Autodesk Inventor part; units mm, degrees
ref_plane "YZ Plane" through (0, 0, 0) normal (1, 0, 0) x (0, 1, 0)
ref_plane "XZ Plane" through (0, 0, 0) normal (0, 1, 0) x (-1, 0, 0)
ref_plane "XY Plane" through (0, 0, 0) normal (0, 0, 1) x (1, 0, 0)
sketch "Sketch1" plane through (0, 0, 0) normal (0, 0, 1) x (1, 0, 0)
  line L0 (0, 0) -> (25.4, 0)
  line L1 (25.4, 0) -> (25.4, 50.8)
  line L2 (25.4, 50.8) -> (0, 50.8)
  line L3 (0, 50.8) -> (0, 0)
  line L4 (1.5875, 49.2125) -> (23.8125, 49.2125)
  line L5 (23.8125, 49.2125) -> (23.8125, 1.5875)
  line L6 (23.8125, 1.5875) -> (1.5875, 1.5875)
  line L7 (1.5875, 1.5875) -> (1.5875, 49.2125)
  dimension "d0" = 25.4
  dimension "d1" = 50.8
  dimension "d2" = 1.5875
extrude "Extrusion1" add sketch "Sketch1" along normal blind 76.2
sketch "Sketch2" plane through (25.4, 0, 0) normal (1, 0, 0) x (0, 0, -1)
  circle A0 centre (-38.1, 25.4) radius 7.9375
  point P0 (0, 0)
  dimension "d5" = 15.875
extrude "Extrusion2" cut sketch "Sketch2" against normal blind 4.7625
sketch "Sketch3" plane through (0, 0, 0) normal (-1, 0, 0) x (0, 0, 1)
  circle A0 centre (38.1, 25.4) radius 7.9375
  circle A1 centre (38.1, 25.4) radius 6.35
  point P0 (0, 0)
  dimension "d8" = 12.7
extrude "Extrusion3" cut sketch "Sketch3" against normal blind 4.7625 contours A1
sketch "Sketch4" plane through (0, 0, 0) normal (-1, 0, 0) x (0, 0, 1)
  line L0 (0, 1.5875) -> (0, 49.2125) construction
  line L1 (0, 25.4) -> (12.7, 25.4) construction
  line L2 (12.7, 25.4) -> (63.5, 25.4) construction
  circle A0 centre (12.7, 25.4) radius 2.5797
  circle A1 centre (63.5, 25.4) radius 2.5797
  point P0 (0, 0)
  dimension "d11" = 12.7
  dimension "d12" = 50.8
  dimension "d13" = 5.1594
extrude "Extrusion4" cut sketch "Sketch4" against normal blind 55.5625
sketch "Sketch5" plane through (0, 50.8, 0) normal (0, 1, 0) x (1, 0, 0)
  line L0 (23.8125, 0) -> (1.5875, 0) construction
  line L1 (12.7, 0) -> (12.7, -12.7) construction
  line L2 (12.7, -12.7) -> (12.7, -63.5) construction
  circle A0 centre (12.7, -12.7) radius 2.5797
  circle A1 centre (12.7, -63.5) radius 2.5797
  point P0 (0, 0)
  dimension "d16" = 12.7
  dimension "d17" = 50.8
  dimension "d18" = 5.1594
extrude "Extrusion5" cut sketch "Sketch5" against normal blind 66.675
properties part number "new piston mount v1"
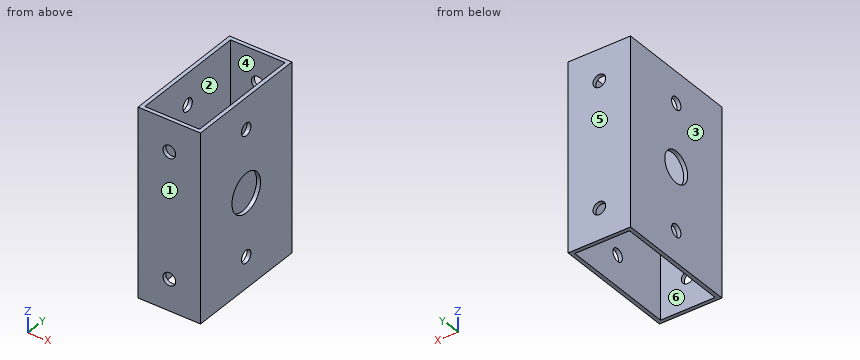
Source: CAD feature listing. Evaluate the final solid. Frame: model axes, mm. Face numbers are marked on the shaded views. A direction names the side the tool comes from. Coordinates: 2 decimals unless noted, no trailing zeros. Loops run counter-clockwise (first coordinate to the right, second up) from the corner with the lowest first, then second, coordinate; pieces in that order, holes last. Notation, with made-up numbers: M 82.5,61 L 87.5,61 A28 ccw 87.5,88 Z; hole C -37.75,-36 d5. An arc over 180 degrees is marked long. Put each result on its own line as item: value. Start each with the question number.
1) Cut plane C-C on z = 48.5. Return the cut outline in (x, y).
2) Ray query, L1, parallel to Z at x = 12.7, y = 0.45; L2, parallel to X at y = 33, z = 5.5; L3, parallel to Y at x = 23.5, z = 31.5. Return the intervals inside material, ascending. Write a range as from..to.
3) Cut plane D-D on y = 16. Return the cut outline in (x, z).
4) Cut plane B-B on y = 25.4. Give the number of separate pieces and of enclosed holes in the cut face, then the cut area to 3 significant figures.
5) Reachability of the marked faces 1 and 2 from +Z, -Z, +X, -X, +Y, -Y: full face, straight path, thin tool, end or side. Return the list, or none.
6) Cut plane A-A on x = 12.7. Return the cut outline in (y, z).
7) Pull-direction query (X, two-part tool) for the marked faces 3, 4, 5 and 6; classes: pulls with the +X half, pulls with the -X half, needs draft (parallel to the pull), parting line crosses it, or undercut.
8) Contact query for a flat-ended pin moving along its axis: pin 1 Ø3 at (y, z) = (25.4, 63.5) entering from +X. Output: stop coordinate, or through.
The answers:
1. outline: M 0,0 L 25.4,0 L 25.4,50.8 L 0,50.8 Z; hole M 1.59,1.59 L 23.81,1.59 L 23.81,49.21 L 1.59,49.21 Z
2. L1: z = 0..10.12, 15.28..60.92, 66.08..76.2
2. L2: x = 0..1.59, 23.81..25.4
2. L3: y = 0..1.59, 49.21..50.8
3. outline: M 0,0 L 1.59,0 L 1.59,76.2 L 0,76.2 Z; M 23.81,0 L 25.4,0 L 25.4,76.2 L 23.81,76.2 Z
4. separate pieces: 8
4. enclosed holes: 0
4. area: 164 mm²
5. face 1: +Z, -Z, +X, -X, -Y
5. face 2: +Z, -Z
6. outline: M 0,0 L 1.59,0 L 1.59,10.12 L 0,10.12 Z; M 0,15.28 L 1.59,15.28 L 1.59,60.92 L 0,60.92 Z; M 0,66.08 L 1.59,66.08 L 1.59,76.2 L 0,76.2 Z; M 49.21,0 L 50.8,0 L 50.8,10.12 L 49.21,10.12 Z; M 49.21,15.28 L 50.8,15.28 L 50.8,60.92 L 49.21,60.92 Z; M 49.21,66.08 L 50.8,66.08 L 50.8,76.2 L 49.21,76.2 Z
7. face 3: pulls with the -X half
7. face 4: undercut
7. face 5: needs draft
7. face 6: undercut
8. pin 1: passes through
